from build123d import *

# Parameters (mm, degrees)
F0_W      = 80.587271601
F0_H      = 134.6200034022
F1_DEPTH  = 50.8
F3_W      = 22.1672728658
F3_H      = 134.6200034022
F4_DEPTH  = 12.7
F5_DEPTH  = 80.588271601
F6_R      = 7.4930236149
F7_DEPTH  = 81.0970184176
F8_R      = 7.092028965
F9_DEPTH  = 81.0970184176
F10_R     = 7.1305147712
F11_DEPTH = 81.0970184176
F12_R     = 6.445813808
F13_DEPTH = 81.0970184176
F15_DEPTH = 12.7
F16_W     = 62.6918235794
F16_H     = 9.051089175
F17_DEPTH = 80.588271601


with BuildPart() as f1:
    # F0 (on Top) → F1 (new body)
    with BuildSketch(Plane.XY):
        with Locations((0.5772728473, 0.2309121192)):
            Rectangle(F0_W, F0_H)
    extrude(amount=F1_DEPTH)

    # F3 (on face) → F4 (cut)
    with BuildSketch(Plane.XY.offset(50.8)):
        with Locations((9.313e-07, 0.2309121192)):
            Rectangle(F3_W, F3_H)
    extrude(amount=-F4_DEPTH, mode=Mode.SUBTRACT)

    # F2 (on face) → F5 (cut, through all)
    with BuildSketch(Plane(origin=(-39.7163629532, 0, 0), x_dir=(0, -1, 0), z_dir=(-1, 0, 0))):
        Polygon((67.079089582, 50.8), (-0.2309121192, 50.8), (67.079089582, 0), align=None)
    extrude(amount=-F5_DEPTH, mode=Mode.SUBTRACT)

    # F6 (on face) → F7 (cut, through all)
    with BuildSketch(Plane(origin=(0, -24.3426037367, 32.2539507662), x_dir=(1, 0, 0), z_dir=(0, -0.6024068962, 0.7981891577))):
        with Locations((-8.0818189308, -6.697748322)):
            Circle(F6_R)
    extrude(amount=-F7_DEPTH, mode=Mode.SUBTRACT)

    # F8 (on face) → F9 (cut, through all)
    with BuildSketch(Plane(origin=(0, -24.3426037367, 32.2539507662), x_dir=(1, 0, 0), z_dir=(0, -0.6024068962, 0.7981891577))):
        with Locations((-7.3890909553, -32.5778611004)):
            Circle(F8_R)
    extrude(amount=-F9_DEPTH, mode=Mode.SUBTRACT)

    # F10 (on face) → F11 (cut, through all)
    with BuildSketch(Plane(origin=(0, -24.3426037367, 32.2539507662), x_dir=(1, 0, 0), z_dir=(0, -0.6024068962, 0.7981891577))):
        with Locations((25.1690894365, -5.9982873499)):
            Circle(F10_R)
    extrude(amount=-F11_DEPTH, mode=Mode.SUBTRACT)

    # F12 (on face) → F13 (cut, through all)
    with BuildSketch(Plane(origin=(0, -24.3426037367, 32.2539507662), x_dir=(1, 0, 0), z_dir=(0, -0.6024068962, 0.7981891577))):
        with Locations((26.3236388564, -31.878400594)):
            Circle(F12_R)
    extrude(amount=-F13_DEPTH, mode=Mode.SUBTRACT)

    # F14 (on face) → F15 (cut)
    with BuildSketch(Plane(origin=(-39.7163629532, 0, 0), x_dir=(0, -1, 0), z_dir=(-1, 0, 0))):
        Polygon((67.079089582, 0), (19.1769771332, 36.1525367835), (19.1769771332, 0), align=None)
    extrude(amount=-F15_DEPTH, mode=Mode.SUBTRACT)

    # F16 (on face) → F17 (cut, through all)
    with BuildSketch(Plane(origin=(-39.7163629532, 0, 0), x_dir=(0, -1, 0), z_dir=(-1, 0, 0))):
        with Locations((-36.1950020306, 4.5255445875)):
            Rectangle(F16_W, F16_H)
    extrude(amount=-F17_DEPTH, mode=Mode.SUBTRACT)


solid = f1.part
Could you check a few things on this model? Use its own coordinates, in mm. A direction names the side the tool comes from. Give positions to 0.01 mm unless a question says otherwise; leave off trailing zeros. Order: outer loops, then holes, each group sorted by start corner. A loop starts at its lowest first (then second) coordinate and runs counter-clockwise, first axis right, second up. Notation, with made-up numbers: (31.25, 79.25) -> (57.25, 79.25) arc R10 cw to (57.25, 97.25) -> close; hole circle Ø9 at (34.25, 43). An arc over 180 degrees is marked (long way). Answer in a Markdown table with one row per item. Add a question column.
Item 1: Imagine slicing it at D-D (x = -34). List the corners of the cut face in (y, z) for me.
Item 2: Imagine slicing it at A-A (x = -5). List the corners of the cut face in (y, z) for me, and give its area (3 significant figures).
Item 3: Imagine slicing it at B-B (y = 15.5). List the corners of the cut face in (x, z) for me.
Item 4: Please list where these lines run through material, in increasing order: probe 1 along X at (y, z) = (20, 44); probe 2 along Z at (x, y) = (28, 51); probe 3 along Y at (x, z) = (-33, 35.5).
Item 5: We'd pull the mould along Z, two halves only. Please class faces 1 (the flat face through (-26, 34, 50.8)), 2 (the cylindrical face through (25.485, -39.806, 10.434)), 3 (the flat face through (-27.016, -32, 10)): pulls with the +Z half, pulls with the -Z half, needs draft (parallel to the pull), parting line crosses it, or undercut.
Item 6: For faces 4 (the flat face through (-33, -19.177, 18)), 5 (the flat face through (11.084, 25, 45)), 6 (the flat face through (0, 37, 9.051)), which set-ups out of +Z, -Z, +X, -X, +Y, -Y let a thin tool reach every point of the face, with its end or its side?
Item 7: Imagine slicing it at C-C (z = 47.5). List the corners of the cut face in (x, y) for me.
Item 8: I'm going to push flat-ended pins straight in: P1, Ø3, axis at x = -6.5, y = -38.5, coming from the -Z side; P2, Ø19, axis at x = -12.5, y = 45, coming from the -Z side; P3, Ø12, axis at x = 2.5, z = 26, coming from the -Y side; P4, Ø17.5, axis at x = -4.5, y = 22, coming from the +Z side. Where does each tip first touch, or does it pass through?
Result:
| question | item | result |
|---|---|---|
| 1 | outline | (-19.18, 0) -> (4.85, 0) -> (4.85, 9.05) -> (67.54, 9.05) -> (67.54, 50.8) -> (0.23, 50.8) -> (-19.18, 36.15) -> close |
| 2 | outline | (-67.08, 0) -> (-49.18, 0) -> (-55.68, 8.61) -> close; (-45.02, 16.65) -> (-32.45, 0) -> (-16.95, 0) -> (-35.14, 24.1) -> close; (-24.24, 32.33) -> (0.17, 0) -> (4.85, 0) -> (4.85, 9.05) -> (67.54, 9.05) -> (67.54, 38.1) -> (-16.6, 38.1) -> close |
| 2 | area | 2,910 mm2 |
| 3 | outline | (-39.72, 9.05) -> (40.87, 9.05) -> (40.87, 50.8) -> (11.08, 50.8) -> (11.08, 38.1) -> (-11.08, 38.1) -> (-11.08, 50.8) -> (-39.72, 50.8) -> close |
| 4 | probe 1 | -39.72 to -11.08, 11.08 to 40.87 |
| 4 | probe 2 | 9.05 to 50.8 |
| 4 | probe 3 | -19.18 to 67.54 |
| 5 | face 1 | pulls with the +Z half |
| 5 | face 2 | undercut |
| 5 | face 3 | needs draft |
| 6 | face 4 | +Z, -Z, -X, -Y |
| 6 | face 5 | +Z, +Y, -Y |
| 6 | face 6 | -Z, +X, -X, +Y |
| 7 | outline | (-39.72, -4.14) -> (-11.08, -4.14) -> (-11.08, 67.54) -> (-39.72, 67.54) -> close; (11.08, -4.14) -> (40.87, -4.14) -> (40.87, 67.54) -> (11.08, 67.54) -> close |
| 8 | P1 | z = 6.59 |
| 8 | P2 | z = 9.05 |
| 8 | P3 | y = -40.58 |
| 8 | P4 | z = 50.8 |
